```python
from build123d import *

# Parameters (mm, degrees)
F0_R          = 7.25
F1_DEPTH      = 2
F4_W          = 2
F4_H          = 2
F2_DEPTH      = 25
F2_DEPTH_BACK = 25
F3_R          = 4.15
F5_DEPTH      = 25


with BuildPart() as f1:
    # F0 (on Top) → F1 (new body)
    with BuildSketch(Plane.XY):
        Circle(F0_R)
    extrude(amount=F1_DEPTH)

    # F4 (on Front) → F2 (join, two sides)
    with BuildSketch(Plane.XZ) as f2_sk:
        with Locations((0, 1)):
            Rectangle(F4_W, F4_H)
    extrude(amount=F2_DEPTH)
    extrude(f2_sk.sketch, amount=-F2_DEPTH_BACK)

    # F3 (on face) → F5 (cut)
    with BuildSketch(Plane(origin=(0, 0, 0), x_dir=(1, 0, 0), z_dir=(0, 0, -1))):
        Circle(F3_R)
    extrude(amount=-F5_DEPTH, mode=Mode.SUBTRACT)


solid = f1.part
```
CAD build for the part. Positions are in the model's coordinates, mm. A direction names the side the tool comes from. Coordinates: 2 decimals unless noted, no trailing zeros. Write each loop counter-clockwise with the first axis right and the second up, starting at its lowest first coordinate (ties: lowest second). Pieces come first, ordered by that corner, then holes.
(1) Cut at C-C, the plane x = 3.25. List the corners of the cut face in (y, z), and give its area (3 significant figures).
(2) Cut at A-A, the plane y = 0. List the corners of the cut face in (x, z).
(3) 3-axis set-ups, long thin cutter, end or side, ignore diameter. For faces 1 (the face through (-1, 16, 1)), 2 (the face through (1, -16, 1)), 3 (the face through (-2, 4, 0)), 4 (the face through (-1, -16, 1)), 5 (the face through (1, 16, 1)): which of +Z, -Z, +X, -X, +Y, -Y reach the whole face in a straight line?
(4) Cut at D-D, the plane y = 9. List the corners of the cut face in (x, z).
(5) Drill centre lines: probe 1 along Y at (x, z) = (0, 1.05); probe 2 along X at (y, z) = (20.5, 1.8); probe 3 along Y at (x, z) = (-1.75, 1.6). Where is each one in solid material? Low to high.
(6) Cut at B-B, the plane z = 0.45. List the corners of the cut face in (x, y).
(7) Two-plate mould, pull along Y, no slides. Class faces 6 (the face through (0, 25, 1)), 7 (the face through (-2, -4, 2)), 8 (the face through (-0.9, 4.05, 0.99)), 9 (the face through (-7.25, 0.15, 0.99)): +Y half, -Y half, draft (parallel to the pull), parting line (faces both ways), or undercut.
(8) Flat gauge pins, fed straight in: pin 1 (0.6 mm diameter, centred on y = 16, z = 1, fed in from +X); pin 2 (1 mm diameter, centred on x = -5, z = 1.5, fed in from -Y). Where does each tip first touch, or does it go through?
Geometry says:
1. outline: (-6.48, 0) - (-2.58, 0) - (-2.58, 2) - (-6.48, 2) - close; (2.58, 0) - (6.48, 0) - (6.48, 2) - (2.58, 2) - close
1. area: 15.6 mm2
2. outline: (-7.25, 0) - (-4.15, 0) - (-4.15, 2) - (-7.25, 2) - close; (4.15, 0) - (7.25, 0) - (7.25, 2) - (4.15, 2) - close
3. face 1: +Z, -Z, -X, +Y
3. face 2: +Z, -Z, +X, -Y
3. face 3: -Z, +X, -X, +Y, -Y
3. face 4: +Z, -Z, -X, -Y
3. face 5: +Z, -Z, +X, +Y
4. outline: (-1, 0) - (1, 0) - (1, 2) - (-1, 2) - close
5. probe 1: y = -25 to -4.15, 4.15 to 25
5. probe 2: x = -1 to 1
5. probe 3: y = -7.04 to -3.76, 3.76 to 7.04
6. outline: (-1, -25) - (1, -25) - (1, -7.18) arc R7.25 ccw to (1, 7.18) - (1, 25) - (-1, 25) - (-1, 7.18) arc R7.25 ccw to (-1, -7.18) - close; hole circle Ø8.3 at (0, 0)
7. face 6: +Y half
7. face 7: draft
7. face 8: undercut
7. face 9: parting line
8. pin 1: stops at x = 1
8. pin 2: stops at y = -5.68
